Read the model definition and answer for the solid it produces. Units are mm, in the model's axes. A direction names the side the tool comes from. Give positions to 0.01 mm unless a question says otherwise; leave off trailing zeros. Order: outer loops, then holes, each group sorted by start corner. A loop starts at its lowest first (then second) coordinate and runs counter-clockwise, first axis right, second up. Notation, with made-up numbers: M -28,83 L 26,83 A13 cw 26,108 Z; hole C 56,25.25 d5. An arc over 180 degrees is marked long. One line per item, written item: value.
from build123d import *

# Parameters (mm, degrees)
SKETCH_W        = 72.78
SKETCH_H        = 72.78
PAD_DEPTH       = 3
SKETCH002_R     = 0.825
POCKET_DEPTH    = 3.001
SKETCH004_R     = 1.2
SKETCH004_R_2   = 0.825
PAD003_DEPTH    = 2.5
SKETCH005_R     = 1.27
POCKET002_DEPTH = 3.001
SKETCH009_R     = 1.645
SKETCH009_R_2   = 1.27
PAD006_DEPTH    = 2.5
SKETCH010_R     = 1.225
SKETCH010_R_2   = 1.27
POCKET003_DEPTH = 3.001
SKETCH016_R     = 1.645
SKETCH016_R_2   = 1.27
PAD007_DEPTH    = 2.5
SKETCH041_R     = 1.5
POCKET006_DEPTH = 3.001


with BuildPart() as part:
    # Sketch → Pad (new body)
    with BuildSketch(Plane.XY):
        Rectangle(SKETCH_W, SKETCH_H)
    extrude(amount=PAD_DEPTH)

    # Sketch002 (on Face6 of Pad) → Pocket (cut, through all)
    with BuildSketch(Plane.XY.offset(3)):
        with Locations((-20.32, 33.13)):
            Circle(SKETCH002_R)
        with Locations((20.32, 17.89)):
            Circle(SKETCH002_R)
        with Locations((-20.32, 17.89)):
            Circle(SKETCH002_R)
        with Locations((20.32, 33.13)):
            Circle(SKETCH002_R)
    extrude(amount=-POCKET_DEPTH, mode=Mode.SUBTRACT)

    # Sketch004 → Pad003 (join)
    with BuildSketch(Plane.XY.offset(3)):
        with Locations((-20.32, 33.13)):
            Circle(SKETCH004_R)
        with Locations((-20.32, 33.13)):
            Circle(SKETCH004_R_2, mode=Mode.SUBTRACT)
        with Locations((20.32, 17.89)):
            Circle(SKETCH004_R)
        with Locations((20.32, 17.89)):
            Circle(SKETCH004_R_2, mode=Mode.SUBTRACT)
        with Locations((20.32, 33.13)):
            Circle(SKETCH004_R)
        with Locations((20.32, 33.13)):
            Circle(SKETCH004_R_2, mode=Mode.SUBTRACT)
        with Locations((-20.32, 17.89)):
            Circle(SKETCH004_R)
        with Locations((-20.32, 17.89)):
            Circle(SKETCH004_R_2, mode=Mode.SUBTRACT)
    extrude(amount=PAD003_DEPTH)

    # Sketch005 (on Face5 of Pad003) → Pocket002 (cut, through all)
    with BuildSketch(Plane.XY.offset(3)):
        with Locations((-32.9375, 6.985)):
            Circle(SKETCH005_R)
        with Locations((-32.9375, -6.985)):
            Circle(SKETCH005_R)
        with Locations((-17.0625, 6.985)):
            Circle(SKETCH005_R)
        with Locations((-17.0625, -6.985)):
            Circle(SKETCH005_R)
    extrude(amount=-POCKET002_DEPTH, mode=Mode.SUBTRACT)

    # Sketch009 → Pad006 (join)
    with BuildSketch(Plane.XY.offset(3)):
        with Locations((-32.9375, -6.985)):
            Circle(SKETCH009_R)
        with Locations((-32.9375, -6.985)):
            Circle(SKETCH009_R_2, mode=Mode.SUBTRACT)
        with Locations((-17.0625, -6.985)):
            Circle(SKETCH009_R)
        with Locations((-17.0625, -6.985)):
            Circle(SKETCH009_R_2, mode=Mode.SUBTRACT)
        with Locations((-17.0625, 6.985)):
            Circle(SKETCH009_R)
        with Locations((-17.0625, 6.985)):
            Circle(SKETCH009_R_2, mode=Mode.SUBTRACT)
        with Locations((-32.9375, 6.985)):
            Circle(SKETCH009_R)
        with Locations((-32.9375, 6.985)):
            Circle(SKETCH009_R_2, mode=Mode.SUBTRACT)
    extrude(amount=PAD006_DEPTH)

    # Sketch010 (on Face5 of Pad006) → Pocket003 (cut, through all)
    with BuildSketch(Plane.XY.offset(3)):
        with Locations((-26.765, -12.41)):
            Circle(SKETCH010_R)
        with Locations((-6.445, -12.41)):
            Circle(SKETCH010_R_2)
        with Locations((-6.445, -32.73)):
            Circle(SKETCH010_R_2)
        with Locations((-26.765, -32.73)):
            Circle(SKETCH010_R_2)
    extrude(amount=-POCKET003_DEPTH, mode=Mode.SUBTRACT)

    # Sketch016 → Pad007 (join)
    with BuildSketch(Plane.XY.offset(3)):
        with Locations((-6.445, -12.41)):
            Circle(SKETCH016_R)
        with Locations((-6.445, -12.41)):
            Circle(SKETCH016_R_2, mode=Mode.SUBTRACT)
        with Locations((-26.765, -12.41)):
            Circle(SKETCH016_R)
        with Locations((-26.765, -12.41)):
            Circle(SKETCH016_R_2, mode=Mode.SUBTRACT)
        with Locations((-26.765, -32.73)):
            Circle(SKETCH016_R)
        with Locations((-26.765, -32.73)):
            Circle(SKETCH016_R_2, mode=Mode.SUBTRACT)
        with Locations((-6.445, -32.73)):
            Circle(SKETCH016_R)
        with Locations((-6.445, -32.73)):
            Circle(SKETCH016_R_2, mode=Mode.SUBTRACT)
    extrude(amount=PAD007_DEPTH)

    # Sketch041 → Pocket006 (cut, through all)
    with BuildSketch(Plane.XY.offset(3)):
        with Locations((-32.89, 32.89)):
            Circle(SKETCH041_R)
        with Locations((32.89, 32.89)):
            Circle(SKETCH041_R)
        with Locations((-32.89, -32.89)):
            Circle(SKETCH041_R)
        with Locations((32.89, -32.89)):
            Circle(SKETCH041_R)
    extrude(amount=-POCKET006_DEPTH, mode=Mode.SUBTRACT)


with BuildPart() as part_1:
    # Body placement: moved
    add(part.part.moved(Location((0, 0, 18))))


solid = part_1.part
1) Determine the mould class of faces 1 (the face through (-27.122, -14.016, 22.232)), 2 (the face through (-1, 36.39, 19)) for opening direction X: +X half, -X half, draft (parallel to the pull), parting line (faces both ways), or undercut.
Reported:
face 1: undercut
face 2: draft
2) Find section B-B, the plane z = 21.9. Count the separate pieces of the cut face and the enclosed holes in it, plus the area to 3 significant figures.
Reported:
separate pieces: 12
enclosed holes: 12
area: 37.0 mm^2
3) Find section D-D, the plane x = -32.89. Write down the section's boundary in (y, z).
Reported:
outline: M -36.39,18 L -34.39,18 L -34.39,21 L -36.39,21 Z; M -31.39,18 L -8.25,18 L -8.25,23.5 L -8.63,23.5 L -8.63,21 L -31.39,21 Z; M -5.72,18 L 5.72,18 L 5.72,23.5 L 5.34,23.5 L 5.34,21 L -5.34,21 L -5.34,23.5 L -5.72,23.5 Z; M 8.25,18 L 31.39,18 L 31.39,21 L 8.63,21 L 8.63,23.5 L 8.25,23.5 Z; M 34.39,18 L 36.39,18 L 36.39,21 L 34.39,21 Z
4) Each of these flat-tipped pins is pushed along its axis until it touches: pin 1 Ø1.5 at (x, y) = (-6.445, -32.73) entering from +Z; pin 2 Ø1 at (x, y) = (-20, 8) entering from +Z. Where does it stop, or does it pass through?
Reported:
pin 1: passes through
pin 2: stops at z = 21
5) Find section A-A, the plane y = 17.89. Write down the section's boundary in (x, z) (3 decimals), plus the area to 3 significant figures.
Reported:
outline: M -36.39,18 L -21.145,18 L -21.145,23.5 L -21.52,23.5 L -21.52,21 L -36.39,21 Z; M -19.495,18 L 19.495,18 L 19.495,23.5 L 19.12,23.5 L 19.12,21 L -19.12,21 L -19.12,23.5 L -19.495,23.5 Z; M 21.145,18 L 36.39,18 L 36.39,21 L 21.52,21 L 21.52,23.5 L 21.145,23.5 Z
area: 212 mm^2
6) Which of the six approach directions +Z, -Z, +X, -X, +Y, -Y give full straight-line access (tool end or side, diameter ignored) to faces 3 (the face through (-27.122, -34.336, 22.232)), 4 (the face through (-1, 1, 18))?
Reported:
face 3: +Z
face 4: -Z, +X, -X, +Y, -Y
7) Find section C-C, the plane x = -20.32. Write down the section's boundary in (y, z) (3 decimals), plus the area to 3 significant figures.
Reported:
outline: M -36.39,18 L 17.065,18 L 17.065,23.5 L 16.69,23.5 L 16.69,21 L -36.39,21 Z; M 18.715,18 L 32.305,18 L 32.305,23.5 L 31.93,23.5 L 31.93,21 L 19.09,21 L 19.09,23.5 L 18.715,23.5 Z; M 33.955,18 L 36.39,18 L 36.39,21 L 34.33,21 L 34.33,23.5 L 33.955,23.5 Z
area: 212 mm^2
8) Consider probe 1 along Y at (x, z) = (20.32, 22.65) (3 decimals); probe 2 along Y at (x, z) = (-32.89, 18.9); probe 3 along X at (y, z) = (33.13, 19.5) (3 decimals). Determine where each line is inside the solid, lowest interval first.
Reported:
probe 1: y = 16.69 to 17.065, 18.715 to 19.09, 31.93 to 32.305, 33.955 to 34.33
probe 2: y = -36.39 to -34.39, -31.39 to -8.25, -5.72 to 5.72, 8.25 to 31.39, 34.39 to 36.39
probe 3: x = -36.39 to -34.371, -31.409 to -21.145, -19.495 to 19.495, 21.145 to 31.409, 34.371 to 36.39
